The model under review builds one solid part; all positions refer to its coordinate system, in mm. A direction names the side the tool comes from. Coordinates: 2 decimals unless noted, no trailing zeros. Write each loop counter-clockwise with the first axis right and the second up, starting at its lowest first coordinate (ties: lowest second). Pieces come first, ordered by that corner, then holes.
```python
from build123d import *

# Parameters (mm, degrees)
SKETCH_1_R      = 1.5
EXTRUDE_1_DEPTH = 1.5


with BuildPart() as part:
    # Эскиз1 → Бобышка-Вытянуть1 (new, symmetric)
    # profile 1 of 9: a face of its own
    with BuildSketch(Plane.XY):
        with BuildLine():
            Line((-3.325, 7.495623723), (-3.325, 9.642840608))
            ThreePointArc((-3.325, 9.642840608), (-8.833459119, 5.1), (-10.013444932, -1.941885837))
            Line((-10.013444932, -1.941885837), (-8.153900562, -0.868277394))
            ThreePointArc((-8.153900562, -0.868277394), (-7.101408311, 4.1), (-3.325, 7.495623723))
        make_face()
    # profile 2 of 9: a face of its own
    with BuildSketch(Plane.XY):
        with BuildLine():
            Line((-8.153900562, -0.868277394), (-10.013444932, -1.941885837))
            ThreePointArc((-10.013444932, -1.941885837), (-8.833459119, -5.1), (-6.688444932, -7.700954772))
            Line((-6.688444932, -7.700954772), (-4.828900562, -6.627346329))
            ThreePointArc((-4.828900562, -6.627346329), (-7.101408311, -4.1), (-8.153900562, -0.868277394))
        make_face()
    # profile 3 of 9: a face of its own
    with BuildSketch(Plane.XY):
        with BuildLine():
            ThreePointArc((-6.688444932, -7.700954772), (-8.833459119, -5.1), (-10.013444932, -1.941885837))
            Line((-10.013444932, -1.941885837), (-12.639371993, -3.457965532))
            ThreePointArc((-12.639371993, -3.457965532), (-13.856406461, -8), (-9.314371993, -9.217034468))
            Line((-9.314371993, -9.217034468), (-6.688444932, -7.700954772))
        make_face()
        with Locations((-10.976871993, -6.3375)):
            Circle(SKETCH_1_R, mode=Mode.SUBTRACT)
    # profile 4 of 9: a face of its own
    with BuildSketch(Plane.XY):
        with BuildLine():
            ThreePointArc((-6.688444932, -7.700954772), (0, -10.2), (6.688444932, -7.700954772))
            Line((6.688444932, -7.700954772), (4.828900562, -6.627346329))
            ThreePointArc((4.828900562, -6.627346329), (0, -8.2), (-4.828900562, -6.627346329))
            Line((-4.828900562, -6.627346329), (-6.688444932, -7.700954772))
        make_face()
    # profile 5 of 9: a face of its own
    with BuildSketch(Plane.XY):
        with BuildLine():
            ThreePointArc((6.688444932, -7.700954772), (8.833459119, -5.1), (10.013444932, -1.941885837))
            Line((10.013444932, -1.941885837), (8.153900562, -0.868277394))
            ThreePointArc((8.153900562, -0.868277394), (7.101408311, -4.1), (4.828900562, -6.627346329))
            Line((4.828900562, -6.627346329), (6.688444932, -7.700954772))
        make_face()
    # profile 6 of 9: a face of its own
    with BuildSketch(Plane.XY):
        with BuildLine():
            Line((12.639371993, -3.457965532), (10.013444932, -1.941885837))
            ThreePointArc((10.013444932, -1.941885837), (8.833459119, -5.1), (6.688444932, -7.700954772))
            Line((6.688444932, -7.700954772), (9.314371993, -9.217034468))
            ThreePointArc((9.314371993, -9.217034468), (13.856406461, -8), (12.639371993, -3.457965532))
        make_face()
        with Locations((10.976871993, -6.3375)):
            Circle(SKETCH_1_R, mode=Mode.SUBTRACT)
    # profile 7 of 9: a face of its own
    with BuildSketch(Plane.XY):
        with BuildLine():
            ThreePointArc((10.2, 0), (8.305269412, 5.921359641), (3.325, 9.642840608))
            Line((3.325, 9.642840608), (3.325, 7.495623723))
            ThreePointArc((3.325, 7.495623723), (6.874045388, 4.470738194), (8.2, 0))
            ThreePointArc((8.2, 0), (8.18846703, -0.434750156), (8.153900562, -0.868277394))
            Line((8.153900562, -0.868277394), (10.013444932, -1.941885837))
            ThreePointArc((10.013444932, -1.941885837), (10.153254116, -0.975413168), (10.2, 0))
        make_face()
    # profile 8 of 9: a face of its own
    with BuildSketch(Plane.XY):
        with BuildLine():
            Line((3.325, 7.495623723), (3.325, 9.642840608))
            ThreePointArc((3.325, 9.642840608), (0, 10.2), (-3.325, 9.642840608))
            Line((-3.325, 9.642840608), (-3.325, 7.495623723))
            ThreePointArc((-3.325, 7.495623723), (0, 8.2), (3.325, 7.495623723))
        make_face()
    # profile 9 of 9: a face of its own
    with BuildSketch(Plane.XY):
        with BuildLine():
            Line((3.325, 9.642840608), (3.325, 12.675))
            ThreePointArc((3.325, 12.675), (0, 16), (-3.325, 12.675))
            Line((-3.325, 12.675), (-3.325, 9.642840608))
            ThreePointArc((-3.325, 9.642840608), (0, 10.2), (3.325, 9.642840608))
        make_face()
        with Locations((0, 12.675)):
            Circle(SKETCH_1_R, mode=Mode.SUBTRACT)
    extrude(amount=EXTRUDE_1_DEPTH, both=True)


solid = part.part
```
Item 1: Take a section at D-D, the plane y = -4. Write out the cut boundary in (x, z), plus the area to 3 significant figures.
Solved:
outline: (-13.34, -1.5) - (-7.16, -1.5) - (-7.16, 1.5) - (-13.34, 1.5) - close; (7.16, -1.5) - (13.34, -1.5) - (13.34, 1.5) - (7.16, 1.5) - close
area: 37.1 mm2
Item 2: To check wall thickness, follow line 1 along Y through (x, z) = (0.5, -1.3); line 2 along X through (y, z) = (-6.75, -0.3); line 3 along Y through (x, z) = (11.75, -0.35). State the ranges of each line that lie inside material, in increasing order.
Solved:
line 1: y = -10.19 to -8.18, 8.18 to 11.26, 14.09 to 15.96
line 2: x = -14.28 to -12.42, -9.53 to -4.66, 4.66 to 9.53, 12.42 to 14.28
line 3: y = -9.57 to -7.62, -5.05 to -2.94
Item 3: For pin 1 (0.9 mm diameter, centred on y = 10.5, z = -0.5, fed in from -X) (3 decimals); pin 2 (1.5 mm diameter, centred on y = -4.5, z = 1, fed in from +X), all flat-tipped, find the tip position at first contact; note any pin that passes through.
Solved:
pin 1: stops at x = -3.325
pin 2: stops at x = 14.12
Item 4: Take a section at A-A, the plane x = 0. Write out the cut boundary in (y, z) (3 decimals).
Solved:
outline: (-10.2, -1.5) - (-8.2, -1.5) - (-8.2, 1.5) - (-10.2, 1.5) - close; (8.2, -1.5) - (11.175, -1.5) - (11.175, 1.5) - (8.2, 1.5) - close; (14.175, -1.5) - (16, -1.5) - (16, 1.5) - (14.175, 1.5) - close
Item 5: Take a section at B-B, the plane y = 1.5. Write out the cut boundary in (x, z).
Solved:
outline: (-10.09, -1.5) - (-8.06, -1.5) - (-8.06, 1.5) - (-10.09, 1.5) - close; (8.06, -1.5) - (10.09, -1.5) - (10.09, 1.5) - (8.06, 1.5) - close
Item 6: Machinability: for faces 1 (the face through (3.325, 11, 0)), 2 (the face through (0, 16, 0)), 3 (the face through (-3.325, 11, 0)), 4 (the face through (-8.02, -8.47, -0.02)), 5 (the face through (8.4, -0.9, 1.5)), which of the approach directions +Z, -Z, +X, -X, +Y, -Y give a long, thin tool a straight path to every point of the face, cutting with its end or side? Answer none if there is none.
Solved:
face 1: +Z, -Z, +X, +Y
face 2: +Z, -Z, +Y
face 3: +Z, -Z, -X, +Y
face 4: +Z, -Z, -Y
face 5: +Z, +X, -X, +Y, -Y
Item 7: Take a section at C-C, the plane z = -0.85. Count the separate pieces of the cut face and the enclosed holes in it, plus the area to 3 significant figures.
Solved:
separate pieces: 1
enclosed holes: 4
area: 200 mm2
Item 8: Mouldability with a two-part tool opening along Y and no side actions: class faces 6 (the face through (13.82, -8.06, -0.02)), 7 (the face through (-12.475, -6.272, -0.021)), 8 (the face through (-0.1, -10.2, 0)) as pulls with the +Y half, pulls with the -Y half, needs draft (parallel to the pull), parting line crosses it, or undercut.
Solved:
face 6: parting line crosses it
face 7: undercut
face 8: pulls with the -Y half
